Autodesk Inventor part; units mm, degrees
ref_plane "YZ Plane" through (0, 0, 0) normal (1, 0, 0) x (0, 1, 0)
ref_plane "XZ Plane" through (0, 0, 0) normal (0, 1, 0) x (-1, 0, 0)
ref_plane "XY Plane" through (0, 0, 0) normal (0, 0, 1) x (1, 0, 0)
sketch "Sketch1" plane through (0, 0, 0) normal (1, 0, 0) x (0, 1, 0)
  line L0 (0, 0) -> (0, -76)
  line L1 (0, 0) -> (76, 0) construction
  line L2 (0, -76) -> (-46, -76)
  line L3 (-46, -76) -> (-46, 0)
  line L4 (-46, 0) -> (0, 0)
  dimension "d0" = 76
  dimension "d1" = 90
  dimension "d2" = 46
extrude "Extrusion1" add sketch "Sketch1" along normal blind 2
sketch "Sketch2" plane through (0, 0, 0) normal (-1, 0, 0) x (0, 0, 1)
  line L0 (-76, -46) -> (-76, 0)
  line L1 (-76, 0) -> (-73.12, 0)
  line L2 (-76, 0) -> (0, 0)
  line L3 (-73.12, 0) -> (-73.12, -5)
  line L4 (-73.12, -5) -> (-61.12, -5)
  line L5 (-61.12, -5) -> (-61.12, -28)
  line L6 (-61.12, -28) -> (-73.12, -28)
  line L7 (-73.12, -28) -> (-73.12, -5)
  line L8 (-73.12, -5) -> (-37.52, -5)
  line L9 (-37.52, -5) -> (-1.92, -5)
  line L10 (-1.92, -5) -> (-1.92, -28)
  line L11 (-1.92, -28) -> (-13.92, -28)
  line L12 (-13.92, -28) -> (-13.92, -5)
  line L13 (-37.52, -5) -> (-31.52, -5)
  line L14 (-31.52, -5) -> (-31.52, -28)
  line L15 (-31.52, -28) -> (-43.52, -28)
  line L16 (-43.52, -28) -> (-43.52, -5)
  line L17 (-67.12, -28) -> (-67.12, -30.313)
  line L18 (-67.12, -5) -> (-67.12, -2.687)
  circle A0 centre (-67.12, -2.687) radius 1
  circle A1 centre (-67.12, -30.313) radius 1
  line L19 (-37.52, -28) -> (-37.52, -30.313)
  line L20 (-37.52, -5) -> (-37.52, -2.687)
  line L21 (-7.92, -5) -> (-7.92, -2.687)
  line L22 (-7.92, -28) -> (-7.92, -30.313)
  circle A2 centre (-37.52, -2.687) radius 1
  circle A3 centre (-7.92, -2.687) radius 1
  circle A4 centre (-37.52, -30.313) radius 1
  circle A5 centre (-7.92, -30.313) radius 1
  dimension "d5" = 2.88
  dimension "d6" = 5
  dimension "d7" = 12
  dimension "d8" = 23
  dimension "d9" = 12
  dimension "d10" = 35.6
  dimension "d14" = 35.6
  dimension "d15" = 23
  dimension "d16" = 12
  dimension "d17" = 6
  dimension "d18" = 23
  dimension "d19" = 12
  dimension "d24" = 2.313
  dimension "d25" = 2.313
  dimension "d26" = 2
  dimension "d27" = 2
  dimension "d28" = 2
  dimension "d29" = 2
  dimension "d30" = 2
  dimension "d31" = 2
extrude "Extrusion2" cut sketch "Sketch2" against normal up to surface (2 mm away)
sketch "Sketch11" plane through (2, 0, 0) normal (1, 0, 0) x (0, 0, -1)
  line L0 (0, -46) -> (76, -46)
  line L1 (0, -46) -> (14.5664, -60.5664)
  line L2 (0, -46) -> (20.6, -46) construction
  line L3 (76, -46) -> (61.4336, -60.5664)
  line L4 (76, -46) -> (96.6, -46) construction
  line L5 (61.4336, -60.5664) -> (14.5664, -60.5664)
  point P0 (0, 0)
  dimension "d94" = 20.6
  dimension "d95" = 45
  dimension "d96" = 20.6
  dimension "d97" = 135
extrude "Extrusion9" add sketch "Sketch11" against normal up to surface (2 mm away)
sketch "Sketch14" plane through (2, 0, 0) normal (1, 0, 0) x (0, 0, -1)
  line L0 (1.92, -5) -> (13.92, -5)
  line L1 (1.92, -28) -> (1.92, -5)
  line L2 (13.92, -28) -> (1.92, -28)
  circle A0 centre (7.92, -30.313) radius 1
  line L3 (13.92, -5) -> (13.92, -28)
  circle A1 centre (7.92, -2.687) radius 1
  line L4 (14.92, -29) -> (0.92, -29)
  line L5 (0.92, -29) -> (0.92, -4)
  line L6 (0.92, -4) -> (14.92, -4)
  line L7 (14.92, -4) -> (14.92, -29)
  circle A2 centre (7.92, -2.687) radius 2
  circle A3 centre (7.92, -30.313) radius 2
  point P0 (0, 0)
  point P1 (9.4287, -4)
  point P2 (6.4113, -4)
  point P3 (6.4113, -29)
  point P4 (9.4287, -29)
  dimension "d112" = 1
  dimension "d113" = 1
  dimension "d114" = 1
extrude "Extrusion12" add sketch "Sketch14" along normal blind 14.5
sketch "Sketch15" plane through (2, 0, 0) normal (1, 0, 0) x (0, 0, -1)
  line L0 (31.52, -5) -> (43.52, -5)
  line L1 (43.52, -5) -> (43.52, -28)
  line L2 (31.52, -28) -> (31.52, -5)
  line L3 (43.52, -28) -> (31.52, -28)
  circle A0 centre (37.52, -30.313) radius 1
  circle A1 centre (37.52, -2.687) radius 1
  line L4 (44.52, -29) -> (44.52, -4)
  line L5 (44.52, -4) -> (30.52, -4)
  line L6 (30.52, -4) -> (30.52, -29)
  line L7 (30.52, -29) -> (44.52, -29)
  circle A2 centre (37.52, -2.687) radius 2
  circle A3 centre (37.52, -30.313) radius 2
  point P0 (0, 0)
  point P1 (39.0287, -4)
  point P2 (36.0113, -4)
  point P3 (36.0113, -29)
  point P4 (39.0287, -29)
  dimension "d117" = 1
  dimension "d118" = 1
  dimension "d119" = 1
extrude "Extrusion13" add sketch "Sketch15" along normal blind 17
sketch "Sketch16" plane through (2, 0, 0) normal (1, 0, 0) x (0, 0, -1)
  line L0 (61.12, -5) -> (73.12, -5)
  line L1 (73.12, -5) -> (73.12, -28)
  line L2 (61.12, -28) -> (61.12, -5)
  line L3 (73.12, -28) -> (61.12, -28)
  circle A0 centre (67.12, -30.313) radius 1
  circle A1 centre (67.12, -2.687) radius 1
  line L4 (74.12, -4) -> (60.12, -4)
  line L5 (60.12, -4) -> (60.12, -29)
  line L6 (60.12, -29) -> (74.12, -29)
  line L7 (74.12, -29) -> (74.12, -4)
  circle A2 centre (67.12, -2.687) radius 2
  circle A3 centre (67.12, -30.313) radius 2
  point P0 (0, 0)
  point P1 (65.6113, -29)
  point P2 (68.6287, -29)
  point P3 (68.6287, -4)
  point P4 (65.6113, -4)
  dimension "d134" = 90
  dimension "d136" = 0
  dimension "d122" = 1
  dimension "d123" = 1
  dimension "d124" = 1
extrude "Extrusion14" add sketch "Sketch16" along normal blind 14.5
sketch "Sketch17" plane through (2, 0, 0) normal (1, 0, 0) x (0, 0, -1)
  line L0 (76, 0) -> (0, 0)
  line L1 (38, 0) -> (38, -60.5664)
  line L2 (14.5664, -60.5664) -> (61.4336, -60.5664)
  line L3 (38, -42.813) -> (35, -42.813)
  circle A0 centre (35, -42.813) radius 1
  arc A1 (33.687, -44.3217) -> (33.687, -41.3043) centre (35, -42.813) ccw
  line L4 (35, -42.813) -> (32.687, -42.813)
  line L5 (32.687, -42.813) -> (32.687, -36.813)
  line L6 (32.687, -36.813) -> (9.687, -36.813)
  line L7 (9.687, -36.813) -> (9.687, -48.813)
  line L8 (9.687, -48.813) -> (32.687, -48.813)
  line L9 (9.687, -48.813) -> (32.687, -48.813) construction
  line L10 (32.687, -48.813) -> (32.687, -42.813)
  line L11 (9.687, -42.813) -> (7.374, -42.813)
  circle A2 centre (7.374, -42.813) radius 1
  arc A3 (8.687, -41.3043) -> (8.687, -44.3217) centre (7.374, -42.813) ccw
  line L12 (8.687, -35.813) -> (33.687, -35.813)
  line L13 (33.687, -35.813) -> (33.687, -42.813)
  line L14 (33.687, -42.813) -> (33.687, -49.813)
  line L15 (33.687, -49.813) -> (8.687, -49.813)
  line L16 (8.687, -49.813) -> (8.687, -35.813)
  circle A4 centre (41, -42.813) radius 1
  arc A5 (42.313, -41.3043) -> (42.313, -44.3217) centre (41, -42.813) ccw
  line L17 (43.313, -42.813) -> (43.313, -36.813)
  line L18 (43.313, -36.813) -> (66.313, -36.813)
  line L19 (66.313, -36.813) -> (66.313, -48.813)
  line L20 (66.313, -48.813) -> (43.313, -48.813)
  line L21 (43.313, -48.813) -> (43.313, -42.813)
  circle A6 centre (68.626, -42.813) radius 1
  arc A7 (67.313, -44.3217) -> (67.313, -41.3043) centre (68.626, -42.813) ccw
  line L22 (67.313, -35.813) -> (42.313, -35.813)
  line L23 (42.313, -35.813) -> (42.313, -42.813)
  line L24 (42.313, -42.813) -> (42.313, -49.813)
  line L25 (42.313, -49.813) -> (67.313, -49.813)
  line L26 (67.313, -49.813) -> (67.313, -35.813)
  dimension "d127" = 3
  dimension "d128" = 2
  dimension "d129" = 1
  dimension "d130" = 2.313
  dimension "d131" = 6
  dimension "d132" = 23
  dimension "d133" = 12
  dimension "d134" = 90
  dimension "d135" = 23
  dimension "d136" = 0
  dimension "d137" = 2.313
  dimension "d138" = 2
  dimension "d139" = 1
  dimension "d140" = 1
extrude "Extrusion15" add sketch "Sketch17" along normal blind 14.5 contours A0 L4 L13 A1 L3 | L3 A1 L14 L4 A0 | L14 L15 L16 L11 L7 L8 L10 L4 | L13 L4 L5 L6 L7 L11 L16 L12 | A3 L16 | L23 L24 A5 | L23 L22 L26 L25 L24 | A7 L26
sketch "Sketch18" plane through (2, 0, 0) normal (1, 0, 0) x (0, 0, -1)
  line L0 (9.687, -48.813) -> (32.687, -48.813)
  line L1 (32.687, -48.813) -> (32.687, -36.813)
  line L2 (32.687, -36.813) -> (9.687, -36.813)
  line L3 (9.687, -36.813) -> (9.687, -48.813)
  line L4 (43.313, -36.813) -> (43.313, -48.813)
  line L5 (43.313, -48.813) -> (66.313, -48.813)
  line L6 (66.313, -48.813) -> (66.313, -36.813)
  line L7 (66.313, -36.813) -> (43.313, -36.813)
  circle A0 centre (35, -42.813) radius 1
  circle A1 centre (7.374, -42.813) radius 1
  circle A2 centre (41, -42.813) radius 1
  circle A3 centre (68.626, -42.813) radius 1
  point P0 (0, 0)
extrude "Extrusion16" cut sketch "Sketch18" against normal up to surface (2 mm away)
properties part number "Palm_ServoAttachment"
Input: part model. Units: mm. Frame: model coordinates. A direction names the side the tool comes from. Coordinates: 2 decimals unless noted, no trailing zeros. Loops run counter-clockwise (first coordinate to the right, second up) from the corner with the lowest first, then second, coordinate; pieces in that order, holes last. Notation, with made-up numbers: (-38, -6) - (10, -6) arc R32 cw to (10, 28) - close; hole circle Ø5 at (42, 15.5). An arc over 180 degrees is marked (long way). Answer in a Markdown table with one row per item.
(1) Cut plane A-A on z = -50. Output: boundary loops of the cut face in (x, y), plus the area to 3 significant figures.
Model answer:
| item | result |
|---|---|
| outline | (0, -60.57) - (2, -60.57) - (2, -49.81) - (16.5, -49.81) - (16.5, -48.81) - (0, -48.81) - close; (0, -36.81) - (16.5, -36.81) - (16.5, -35.81) - (2, -35.81) - (2, 0) - (0, 0) - close |
| area | 126 mm² |
(2) Mould query, pull axis Y, two halves, no side actions, for faces 5 (the face through (1, -53, -7)), 6 (the face through (9.148, -32.312, -67.184)), 7 (the face through (8, -48.813, -21)), 8 (the face through (16.5, -17.6, -60.9)). Classes: pulls with the +Y half, pulls with the -Y half, needs draft (parallel to the pull), parting line crosses it, or undercut.
Model answer:
| item | result |
|---|---|
| face 5 | pulls with the -Y half |
| face 6 | undercut |
| face 7 | undercut |
| face 8 | needs draft |
(3) Cut plane C-C on y = -20. Output: boundary loops of the cut face in (x, z).
Model answer:
| item | result |
|---|---|
| outline | (0, -76) - (2, -76) - (2, -74.12) - (16.5, -74.12) - (16.5, -73.12) - (0, -73.12) - close; (0, -61.12) - (16.5, -61.12) - (16.5, -60.12) - (2, -60.12) - (2, -44.52) - (19, -44.52) - (19, -43.52) - (0, -43.52) - close; (0, -31.52) - (19, -31.52) - (19, -30.52) - (2, -30.52) - (2, -14.92) - (16.5, -14.92) - (16.5, -13.92) - (0, -13.92) - close; (0, -1.92) - (16.5, -1.92) - (16.5, -0.92) - (2, -0.92) - (2, 0) - (0, 0) - close |
(4) Material intervals for L1, parallel to Z at x = 7.5, y = -6; L2, parallel to Z at x = 16.25, y = -2.5; L3, parallel to Y at x = 8.5, z = -15, sorted ascending. Write a range as from..to.
Model answer:
| item | result |
|---|---|
| L1 | z = -74.12..-73.12, -61.12..-60.12, -44.52..-43.52, -31.52..-30.52, -14.92..-13.92, -1.92..-0.92 |
| L2 | z = -69.11..-68.1, -66.14..-65.13, -39.51..-38.5, -36.54..-35.53, -9.91..-8.9, -6.94..-5.93 |
| L3 | y = -49.81..-48.81, -36.81..-35.81 |
(5) Cut plane D-D on x = 10.25. Count the separate pieces of the cut face and the enclosed holes in it, plus the area to 3 significant figures.
Model answer:
| item | result |
|---|---|
| separate pieces | 5 |
| enclosed holes | 15 |
| area | 450 mm² |
(6) Cut plane B-B on z = -41. Output: boundary loops of the cut face in (x, y), plus the area to 3 significant figures.
Model answer:
| item | result |
|---|---|
| outline | (0, -60.57) - (2, -60.57) - (2, -44.81) - (16.5, -44.81) - (16.5, -43.81) - (0, -43.81) - close; (0, -41.81) - (16.5, -41.81) - (16.5, -40.81) - (2, -40.81) - (2, -29) - (19, -29) - (19, -28) - (0, -28) - close; (0, -5) - (19, -5) - (19, -4) - (2, -4) - (2, 0) - (0, 0) - close |
| area | 134 mm² |
(7) Set-up query: faces 1 (the face through (9, -16, -14.92)), 2 (the face through (9, -49.813, -55)), 3 (the face through (9, -39, -42.313)), 4 (the face through (9, -47, -33.687)). Return all of +Z, -Z, +X, -X, +Y, -Y with unobstructed straight access to the full face (end or side cutting, diameter ignored); none if empty.
Model answer:
| item | result |
|---|---|
| face 1 | +X, +Y |
| face 2 | +Z, -Z, +X, -Y |
| face 3 | +X |
| face 4 | +X, -Y |
(8) Pin query (flat end, axial travel): P1, Ø3.5, axis at x = 8.5, z = -36.5, coming from the -Y side; P2, Ø4, axis at x = 5, z = -19, coming from the -Y side; P3, Ø3.5, axis at x = 7, z = -10.5, coming from the +Y side. Return the tip coordinate at first contact, or that it passes through.
Model answer:
| item | result |
|---|---|
| P1 | stops at y = -44.81 |
| P2 | stops at y = -49.81 |
| P3 | stops at y = -0.87 |
